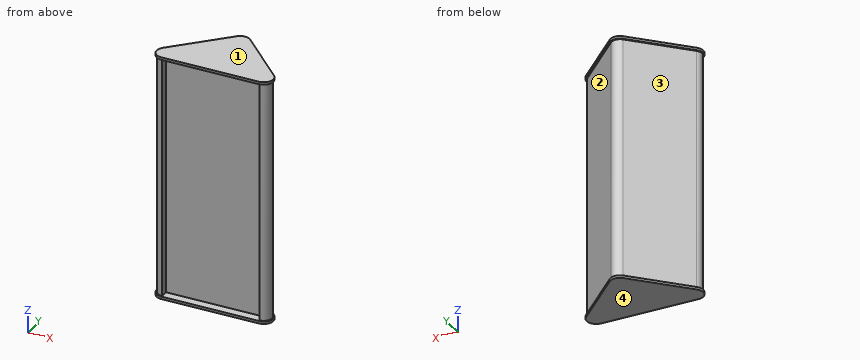
from build123d import *

# Parameters (mm, degrees)
F1_DEPTH    = 4
F2_R        = 15
F4_DEPTH    = 380
F5_T1_DEPTH = 458.4619407771
F5_T3_DEPTH = 412.5
F7_DEPTH    = 4
F8_R        = 15
F9_W        = 153.8477631085
F9_H        = 380
F10_DEPTH   = 12


# Not quite as in the source:
# - a fillet or chamfer that OpenCascade refuses, or shapes differently, is made with other operations: its cross-section is extruded or revolved along the edge and cut away or added


with BuildPart() as f1:
    # F0 (on Top) → F1 (new body)
    with BuildSketch(Plane.XY):
        Polygon((0, 63.1370849898), (-113.1370849898, -50), (113.1370849898, -50), align=None)
    extrude(amount=F1_DEPTH)

    # F2
    f2_edges = [f1.edges().sort_by_distance(p)[0] for p in [
        (-113.137085, -50, 2),
        (113.137085, -50, 2),
        (0, 63.137085, 2),
    ]]
    fillet(f2_edges, radius=F2_R)

    # F3 (on face) → F4 (join)
    with BuildSketch(Plane.XY.offset(4)):
        Polygon((108.3086578651, -48), (0, 60.3086578651), (-108.3086578651, -48), align=None)
    extrude(amount=F4_DEPTH)

    # F5: fillet of radius 13 on 3 edges, made by hand

    # F5_s2 → F5_t1 (cut)
    with BuildSketch(Plane.XY.offset(4)):
        with BuildLine():
            ThreePointArc((86.1162697097, -25.8076118446), (88.9343154769, -39.9748846207), (76.9238815543, -48))
            Line((76.9238815543, -48), (108.3086578651, -48))
            Line((108.3086578651, -48), (86.1162697097, -25.8076118446))
        make_face()
        with BuildLine():
            ThreePointArc((-86.1162697097, -25.8076118446), (-88.9343154769, -39.9748846207), (-76.9238815543, -48))
            Line((-76.9238815543, -48), (-108.3086578651, -48))
            Line((-108.3086578651, -48), (-86.1162697097, -25.8076118446))
        make_face()
    extrude(amount=F5_T1_DEPTH, mode=Mode.SUBTRACT)

    # F5_s4 → F5_t3 (cut)
    with BuildSketch(Plane.XY.offset(4)):
        with BuildLine():
            ThreePointArc((-9.1923881554, 51.1162697097), (0, 54.9238815543), (9.1923881554, 51.1162697097))
            Line((9.1923881554, 51.1162697097), (0, 60.3086578651))
            Line((0, 60.3086578651), (-9.1923881554, 51.1162697097))
        make_face()
    extrude(amount=F5_T3_DEPTH, mode=Mode.SUBTRACT)

    # F6 (on face) → F7 (join)
    with BuildSketch(Plane.XY.offset(384)):
        Polygon((0, 63.1370849898), (-113.1370849898, -50), (113.1370849898, -50), align=None)
    extrude(amount=F7_DEPTH)

    # F8
    f8_edges = [f1.edges().sort_by_distance(p)[0] for p in [
        (113.137085, -50, 386),
        (-113.137085, -50, 386),
        (0, 63.137085, 386),
    ]]
    fillet(f8_edges, radius=F8_R)

    # F9 (on face) → F10 (cut)
    with BuildSketch(Plane.XZ.offset(48)):
        with Locations((0, 194)):
            Rectangle(F9_W, F9_H)
    extrude(amount=-F10_DEPTH, mode=Mode.SUBTRACT)


solid = f1.part
Source: CAD feature listing. Evaluate the final solid. Frame: model axes, mm. Face numbers are marked on the shaded views. Round coordinates to 2 decimals unless told otherwise and drop trailing zeros. Loops run counter-clockwise (first coordinate to the right, second up) from the corner with the lowest first, then second, coordinate; pieces in that order, holes last. Notation, with made-up numbers: M 63,63.25 L 96,63.25 A8 ccw 96,77.25 Z; hole C 13,53.25 d2. An arc over 180 degrees is marked long. Return JSON: item names as keys, results as strings. Group by question number.
1. Material intervals for line 1 along Z through (x, y) = (48.5, -43); line 2 along X through (y, z) = (-42.5, 53.5); line 3 along Y through (x, z) = (-56, 70.5), sorted ascending. Write a range as from..to.
2. Section query B-B on z = 261.5. Output: boundary loops of the cut face in (x, y).
3. Mould query, pull axis Z, two halves, no side actions, for the marked faces 1, 2, 3 and 4. Classes: released by +Z, released by -Z, zero draft, split by the parting line, or undercut.
4. Section query C-C on x = 23. Output: boundary loops of the cut face in (y, z), and give its area (3 significant figures).
5. Pin query (flat end, axial travel): pin 1 (9.5 mm diameter, centred on y = -41.5, z = 223.5, fed in from +X); pin 2 (8 mm diameter, centred on x = 30, z = 203, fed in from +Y); pin 3 (6 mm diameter, centred on x = -64, z = 172, fed in from -Y); pin 4 (8 mm diameter, centred on x = 23.5, y = -4.5, fed in from -Z). Return the tip coordinate at first contact, or that it passes through.
6. Section query A-A on y = 7. Output: boundary loops of the cut face in (x, z), and give its area (3 significant figures).
Checks:
{
 "1": {"line 1": "z = 0..4, 384..388", "line 2": "x = -87.54..-76.92, 76.92..87.54", "line 3": "y = -36..4.31"},
 "2": {"outline": "M -86.12,-25.81 A13 ccw -76.92,-48 L -76.92,-36 L 76.92,-36 L 76.92,-48 A13 ccw 86.12,-25.81 L 9.19,51.12 A13 ccw -9.19,51.12 Z"},
 "3": {"face 1": "released by +Z", "face 2": "undercut", "face 3": "undercut", "face 4": "released by -Z"},
 "4": {"outline": "M -50,0 L 40.14,0 L 40.14,4 L 37.31,4 L 37.31,384 L 40.14,384 L 40.14,388 L -50,388 L -50,384 L -36,384 L -36,4 L -50,4 Z", "area": "28,600 mm²"},
 "5": {"pin 1": "stops at x = 89.81", "pin 2": "stops at y = 34.31", "pin 3": "stops at y = -36", "pin 4": "stops at z = 0"},
 "6": {"outline": "M -56.14,0 L 56.14,0 L 56.14,4 L 53.31,4 L 53.31,384 L 56.14,384 L 56.14,388 L -56.14,388 L -56.14,384 L -53.31,384 L -53.31,4 L -56.14,4 Z", "area": "41,400 mm²"}
}
